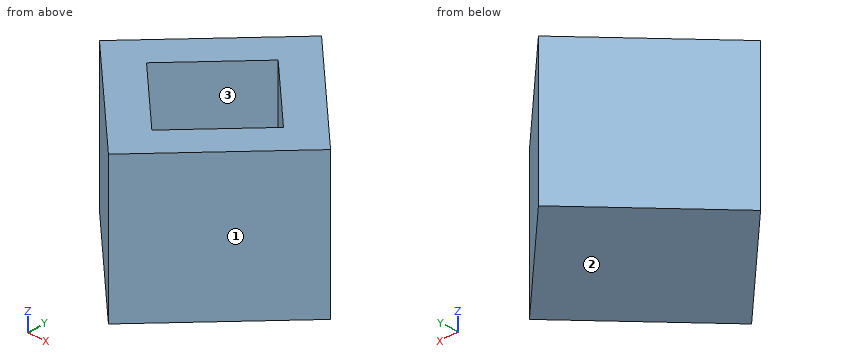
Autodesk Inventor part; units mm, degrees
ref_plane "YZ Plane" through (0, 0, 0) normal (1, 0, 0) x (0, 1, 0)
ref_plane "XZ Plane" through (0, 0, 0) normal (0, 1, 0) x (-1, 0, 0)
ref_plane "XY Plane" through (0, 0, 0) normal (0, 0, 1) x (1, 0, 0)
sketch "Sketch1" plane through (0, 0, 0) normal (0, 0, 1) x (1, 0, 0)
  line L0 (13.4704, 0) -> (0, -13.4704)
  line L1 (0, -13.4704) -> (-13.4704, 0)
  line L2 (-13.4704, 0) -> (0, 13.4704)
  line L3 (0, 13.4704) -> (13.4704, 0)
  line L4 (0, 0) -> (0, 13.4704) construction
  dimension "d0" = 19.05
extrude "Extrusion1" add sketch "Sketch1" against normal blind 16.9333
sketch "Sketch2" plane through (0, 0, -16.9333) normal (0, 0, -1) x (-1, 0, 0)
  circle A0 centre (0, 0) radius 4
  dimension "d3" = 8
sketch "Sketch3" plane through (0, 0, 0) normal (0, 0, 1) x (1, 0, 0)
  line L0 (0, 7.9824) -> (7.9824, 0)
  line L1 (7.9824, 0) -> (0, -7.9824)
  line L2 (0, -7.9824) -> (-7.9824, 0)
  line L3 (-7.9824, 0) -> (0, 7.9824)
  line L4 (-7.9824, 0) -> (0, 0) construction
  dimension "d4" = 11.2889
extrude "Extrusion2" cut sketch "Sketch3" against normal blind 8.4667
properties part number "Driver Shaft"
Geometry: final body of the model. Coordinates: model frame, mm. Face numbers are marked on the shaded views. Round coordinates to 2 decimals unless told otherwise and drop trailing zeros. Order: outer loops, then holes, each group sorted by start corner. A loop starts at its lowest first (then second) coordinate and runs counter-clockwise, first axis right, second up. Notation, with made-up numbers: (-27, 48.5) - (22, 48.5) arc R11 ccw to (22, 66.5) - close; hole circle Ø5 at (-27.75, 47.25). An arc over 180 degrees is marked (long way). Use CSV: the item, a comma, the result in double quotes. Start each with the question number.
Q1. Material intervals for line 1 along Z through (x, y) = (2.5, -1); line 2 along X through (y, z) = (-1, -2.5); line 3 along X through (y, z) = (-5, -8), sorted ascending. Write a range as from..to.
Q2. First-contact query: pin 1 (1 mm diameter, centred on x = -8.5, y = 6.5, fed in from +Z); pin 2 (5 mm diameter, centred on x = -7, z = -11, fed in from +Y); pin 3 (1.5 mm diameter, centred on x = 9, z = -7.5, fed in from +Y). Flat tips, straight axial feed; report the tip coordinate or a pass-through.
Q3. Mould query, pull axis X, two halves, no side actions, for the marked faces 1, 2 and 3. Classes: +X half, -X half, draft (parallel to the pull), parting line (faces both ways), or undercut.
Q4. Section query D-D (z = -16). Return loops of the section in (x, y).
Q5. Section query A-A (z = -4.25). Return loops of the section in (x, y).
Q6. Section query C-C (y = -3.5). Return loops of the section in (x, z).
Q7. Section query B-B (x = -4.25). Return loops of the section in (y, z), and give its area (3 significant figures).
Result set:
1,line 1,"z = -16.93..-8.47"
1,line 2,"x = -12.47..-6.98, 6.98..12.47"
1,line 3,"x = -8.47..-2.98, 2.98..8.47"
2,pin 1,"passes through"
2,pin 2,"stops at y = 8.97"
2,pin 3,"stops at y = 5.22"
3,face 1,"+X half"
3,face 2,"draft"
3,face 3,"undercut"
4,outline,"(-13.47, 0) - (0, -13.47) - (13.47, 0) - (0, 13.47) - close"
5,outline,"(-13.47, 0) - (0, -13.47) - (13.47, 0) - (0, 13.47) - close; hole (-7.98, 0) - (0, -7.98) - (7.98, 0) - (0, 7.98) - close"
6,outline,"(-9.97, -16.93) - (9.97, -16.93) - (9.97, 0) - (4.48, 0) - (4.48, -8.47) - (-4.48, -8.47) - (-4.48, 0) - (-9.97, 0) - close"
7,outline,"(-9.22, -16.93) - (9.22, -16.93) - (9.22, 0) - (3.73, 0) - (3.73, -8.47) - (-3.73, -8.47) - (-3.73, 0) - (-9.22, 0) - close"
7,area,"249 mm2"
